Job drawing, mm, ordinate dimensions from the low corner. One solid piece. Coordinates: 2 decimals unless noted, no trailing zeros. Loops run counter-clockwise (first coordinate to the right, second up) from the corner with the lowest first, then second, coordinate; pieces in that order, holes last. Notation, with made-up numbers: M -6.75,82 L 17.25,82 A13 cw 17.25,99 Z; hole C -20,-0.5 d2. An arc over 180 degrees is marked long. Write each question's results on one line, items separated by ' | '. Start each with the question number.
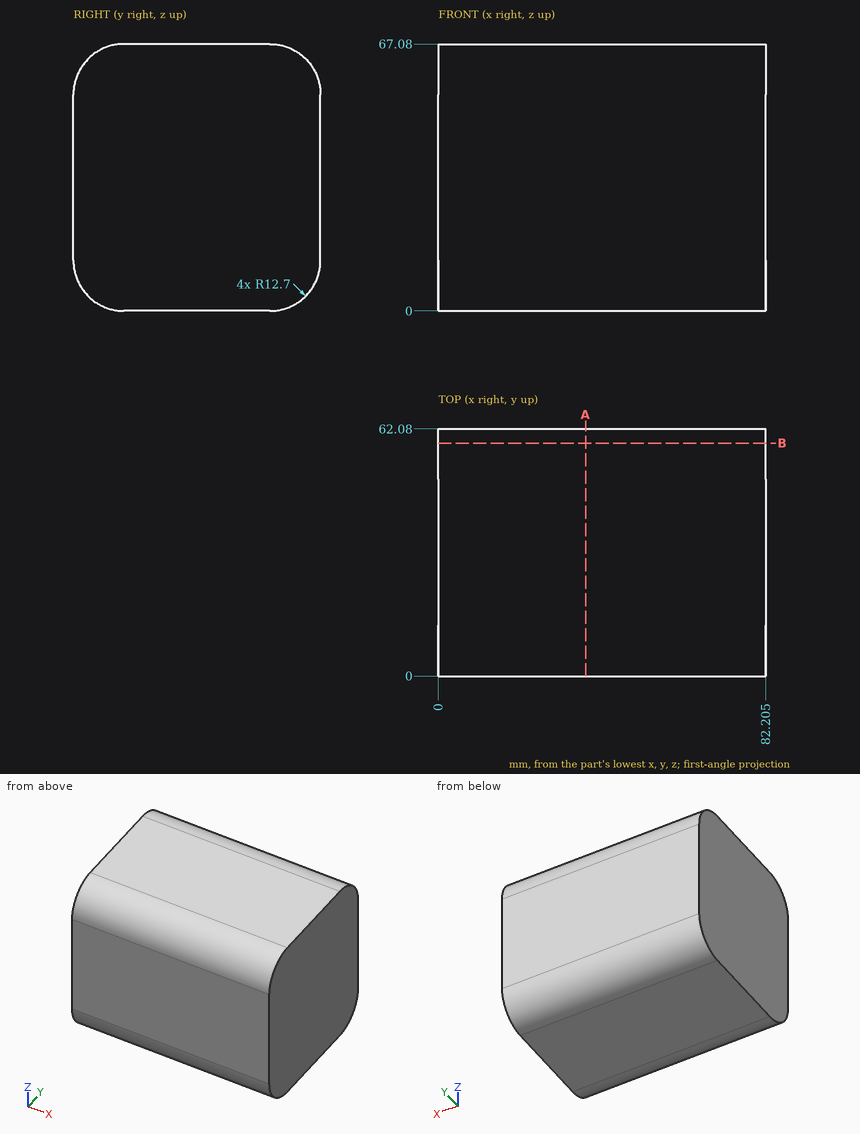
1. Band-saw the part on B-B, the plane y = 58.5. List the corners of the cut face in (x, z) (1 decimal), plus the area to 3 significant figures.
2. Pin check, flat tip, straight feed: pin 1 (3 mm diameter, centred on x = 37, y = 54, fed in from +Z). Stop position of the tip, or through.
3. Band-saw the part on A-A, the plane x = 37. List the corners of the cut face in (y, z).
4. Wall check: line 1 along Z through (x, y) = (52.5, 50) (1 decimal); line 2 along Y through (x, z) = (72, 57); line 3 along Z through (x, y) = (29, 56). Give the ranges that are in metal, low to high.
Checked values:
1) outline: M 0,3.9 L 82.2,3.9 L 82.2,63.2 L 0,63.2 Z | area: 4,880 mm²
2) pin 1: z = 66.69
3) outline: M 0,12.7 A12.7 ccw 12.7,0 L 49.38,0 A12.7 ccw 62.08,12.7 L 62.08,54.38 A12.7 ccw 49.38,67.08 L 12.7,67.08 A12.7 ccw 0,54.38 Z
4) line 1: 0 to 67.1 | line 2: 0.27 to 61.81 | line 3: 1.86 to 65.22
